Could you check a few things on this model? Use its own coordinates, in mm. Face numbers are marked on the shaded views. Give positions to 0.01 mm unless a question says otherwise; leave off trailing zeros. Order: outer loops, then holes, each group sorted by start corner. A loop starts at its lowest first (then second) coordinate and runs counter-clockwise, first axis right, second up. Notation, with made-up numbers: M -4,58 L 50,58 A22 cw 50,77 Z; hole C 36,-6 d1. An arc over 180 degrees is marked long. Use a Markdown table: item, result. Add a question column.
Item 1: Suppose I cut it at D-D on z = 80.5. Write out the boundary of the cut face in (x, y), plus the area to 3 significant figures.
Item 2: Suppose I cut it at A-A on z = 96.5. Write out the boundary of the cut face in (x, y), plus the area to 3 significant figures.
Item 3: I'm going to push flat-ended pins straight in: pin 1 Ø4 at (y, z) = (7, 88) entering from +X; pin 2 Ø2 at (x, z) = (4, 79) entering from -Y; pin 3 Ø6 at (x, z) = (10.5, 58.5) entering from +Y. Where does each tip first touch, or does it pass through?
Item 4: Suppose I cut it at C-C on y = -2.5. Write out the boundary of the cut face in (x, z).
Item 5: If we mould it in two halves opening along X, with no side actions, what happens to the marked faces 1, 2, 3 and 4? For each: released by +X, released by -X, zero draft, split by the parting line, or undercut.
Item 6: If I drill on L1, parallel to Y at x = 0, z = 44; L2, parallel to X at y = 8.5, z = 27; L3, parallel to X at y = -16.5, z = 83.5, over which ranges is the centre line in solid material (lowest first)? Write a range as from..to.
Item 7: Suppose I cut it at B-B on x = 0. Write out the boundary of the cut face in (y, z), plus the area to 3 significant figures.
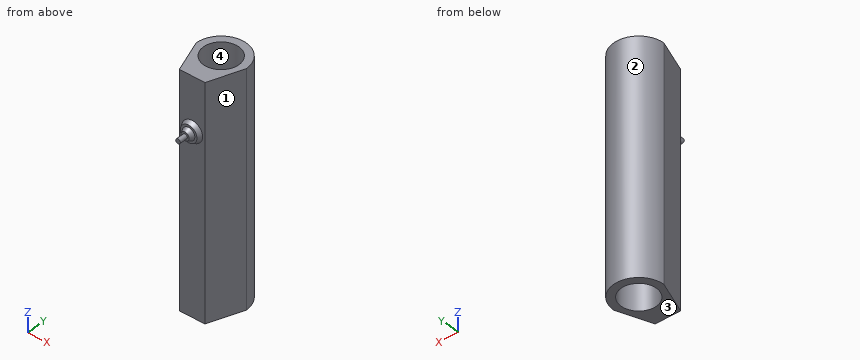
from build123d import *

# Parameters (mm, degrees)
SKETCH1_R  = 9.65
BODY_DEPTH = 125.3


with BuildPart() as part:
    # Sketch1 → Body (new body)
    with BuildSketch(Plane.XY.offset(125.3)):
        with BuildLine():
            Line((-7.016550666, -18.5), (7.016550666, -18.5))
            Line((7.016550666, -18.5), (13.75, 0))
            ThreePointArc((13.75, 0), (0, 13.75), (-13.75, 0))
            Line((-13.75, 0), (-7.016550666, -18.5))
        make_face()
        Circle(SKETCH1_R, mode=Mode.SUBTRACT)
    extrude(amount=-BODY_DEPTH)

    # Sketch2 → Electric-Output (revolve)
    with BuildSketch(Plane(origin=(0, 0, 0), x_dir=(0, 0, -1), z_dir=(1, 0, 0))):
        Polygon((-91.921275864, -20.75), (-90.75, -18.5), (-96.5, -18.5), (-96.5, -23), (-96.5, -27.5), (-95.25, -27.5), (-95.25, -23), (-94.25, -23), (-93.078724136, -20.75), align=None)
    revolve(axis=Axis((0, -23, 96.5), (0, 1, 0)))


solid = part.part
Findings below:
| question | item | result |
|---|---|---|
| 1 | outline | M -13.75,0 L -7.02,-18.5 L 7.02,-18.5 L 13.75,0 A13.75 ccw Z; hole C 0,0 d19.3 |
| 1 | area | 389 mm^2 |
| 2 | outline | M -13.75,0 L -7.02,-18.5 L -5.75,-18.5 L -4.58,-20.75 L -3.42,-20.75 L -2.25,-23 L -1.25,-23 L -1.25,-27.5 L 1.25,-27.5 L 1.25,-23 L 2.25,-23 L 3.42,-20.75 L 4.58,-20.75 L 5.75,-18.5 L 7.02,-18.5 L 13.75,0 A13.75 ccw Z; hole C 0,0 d19.3 |
| 2 | area | 436 mm^2 |
| 3 | pin 1 | stops at x = 12.81 |
| 3 | pin 2 | stops at y = -18.5 |
| 3 | pin 3 | stops at y = 11.52 |
| 4 | outline | M -12.84,0 L -9.32,0 L -9.32,125.3 L -12.84,125.3 Z; M 9.32,0 L 12.84,0 L 12.84,125.3 L 9.32,125.3 Z |
| 5 | face 1 | released by +X |
| 5 | face 2 | split by the parting line |
| 5 | face 3 | zero draft |
| 5 | face 4 | undercut |
| 6 | L1 | y = -18.5..-9.65, 9.65..13.75 |
| 6 | L2 | x = -10.81..-4.57, 4.57..10.81 |
| 6 | L3 | x = -7.74..7.74 |
| 7 | outline | M -27.5,95.25 L -23,95.25 L -23,94.25 L -20.75,93.08 L -20.75,91.92 L -18.5,90.75 L -18.5,0 L -9.65,0 L -9.65,125.3 L -18.5,125.3 L -18.5,102.25 L -20.75,101.08 L -20.75,99.92 L -23,98.75 L -23,97.75 L -27.5,97.75 Z; M 9.65,0 L 13.75,0 L 13.75,125.3 L 9.65,125.3 Z |
| 7 | area | 1,670 mm^2 |
